Could you check a few things on this model? Use its own coordinates, in mm. A direction names the side the tool comes from. Round coordinates to 2 decimals unless told otherwise and drop trailing zeros. Write each loop counter-clockwise with the first axis right and the second up, starting at its lowest first coordinate (ties: lowest second). Pieces come first, ordered by that corner, then holes.
```python
from build123d import *

# Parameters (mm, degrees)
SKETCH1_R               = 0.6
FINGER_PIP_BODY_DEPTH   = 2
FINGER_PIP_CONTOURING_R = 2


with BuildPart() as part:
    # Sketch1 → Finger PIP Body (new body)
    with BuildSketch(Plane.XY):
        with BuildLine():
            Line((0, 6.5), (0, 33.5))
            add(Edge.make_bspline(
                [(0, 33.5), (3.125, 33.9), (6.25, 33.5)],
                knots=[0, 0, 0, 1, 1, 1], degree=2))
            Line((6.25, 33.5), (6.25, 35.5))
            add(Edge.make_bspline(
                [(0, 35.5), (3.125, 35.1), (6.25, 35.5)],
                knots=[0, 0, 0, 1, 1, 1], degree=2))
            Line((0, 35.5), (0, 40))
            Line((0, 40), (20, 40))
            Line((20, 40), (20, 35.5))
            add(Edge.make_bspline(
                [(20, 35.5), (16.875, 35.1), (13.75, 35.5)],
                knots=[0, 0, 0, 1, 1, 1], degree=2))
            Line((13.75, 35.5), (13.75, 33.5))
            add(Edge.make_bspline(
                [(20, 33.5), (16.875, 33.9), (13.75, 33.5)],
                knots=[0, 0, 0, 1, 1, 1], degree=2))
            Line((20, 33.5), (20, 6.5))
            add(Edge.make_bspline(
                [(20, 6.5), (16.875, 6.1), (13.75, 6.5)],
                knots=[0, 0, 0, 1, 1, 1], degree=2))
            Line((13.75, 6.5), (13.75, 4.5))
            add(Edge.make_bspline(
                [(20, 4.5), (16.875, 4.9), (13.75, 4.5)],
                knots=[0, 0, 0, 1, 1, 1], degree=2))
            Line((20, 4.5), (20, 0))
            Line((20, 0), (0, 0))
            Line((0, 0), (0, 4.5))
            add(Edge.make_bspline(
                [(0, 4.5), (3.125, 4.9), (6.25, 4.5)],
                knots=[0, 0, 0, 1, 1, 1], degree=2))
            Line((6.25, 4.5), (6.25, 6.5))
            add(Edge.make_bspline(
                [(0, 6.5), (3.125, 6.1), (6.25, 6.5)],
                knots=[0, 0, 0, 1, 1, 1], degree=2))
        make_face()
        with Locations((3, 2.5)):
            Circle(SKETCH1_R, mode=Mode.SUBTRACT)
        with Locations((5, 9.5)):
            Circle(SKETCH1_R, mode=Mode.SUBTRACT)
        with Locations((5, 30.5)):
            Circle(SKETCH1_R, mode=Mode.SUBTRACT)
        with Locations((3, 37.5)):
            Circle(SKETCH1_R, mode=Mode.SUBTRACT)
        with Locations((17, 37.5)):
            Circle(SKETCH1_R, mode=Mode.SUBTRACT)
        with Locations((15, 30.5)):
            Circle(SKETCH1_R, mode=Mode.SUBTRACT)
        with Locations((15, 9.5)):
            Circle(SKETCH1_R, mode=Mode.SUBTRACT)
        with Locations((17, 2.5)):
            Circle(SKETCH1_R, mode=Mode.SUBTRACT)
    extrude(amount=FINGER_PIP_BODY_DEPTH)

    # Finger PIP Contouring
    finger_pip_contouring_edges = [part.edges().sort_by_distance(p)[0] for p in [
        (0, 40, 1),
        (20, 40, 1),
        (20, 0, 1),
        (0, 0, 1),
    ]]
    fillet(finger_pip_contouring_edges, radius=FINGER_PIP_CONTOURING_R)


solid = part.part
```
Q1. If I drill on L1, parallel to X at y = 37.5, z = 1.15; L2, parallel to Y at x = 17, z = 1.1; L3, parallel to Y at x = 5.25, z = 0.65, over which ranges is the centre line in solid material (lowest first)?
Q2. Imagine slicing it at B-B, the plane x = 15. Count the separate pieces of the cut face and the enclosed holes in it, then the cut area to 3 significant figures.
Q3. I'm going to push flat-ended pins straight in: pin 1 Ø10 at (x, y) = (10.5, 5) entering from -Z; pin 2 Ø1.1 at (x, y) = (3, 2.5) entering from -Z. Where does each tip first touch, or does it pass through?
Q4. Imagine slicing it at A-A, the plane y = 9.5. Write out the boundary of the cut face in (x, z), then the cut area to 3 significant figures.
Q5. We'd pull the mould along Y, two halves only. Please class faces 1 (the flat face through (0, 20, 1)), 2 (the cylindrical face through (14.922, 31.095, 0.986)), 3 (the flat face through (10, 0, 1)): pulls with the +Y half, pulls with the -Y half, needs draft (parallel to the pull), parting line crosses it, or undercut.
Q6. On a 3-axis mill with a long thin cutter (end or side, diameter ignored), from which of +Z, -Z, +X, -X, +Y, -Y can I reach the whole of each face in a straight line? I mean faces 4 (the flat face through (13.75, 35, 1)), 5 (the flat face through (10, 20, 2)). Say none if no direction works.
Results found:
1. L1: x = 0 to 2.4, 3.6 to 16.4, 17.6 to 20
1. L2: y = 0 to 1.9, 3.1 to 4.7, 6.3 to 33.7, 35.3 to 36.9, 38.1 to 40
1. L3: y = 0 to 4.61, 6.39 to 8.95, 10.05 to 29.95, 31.05 to 33.61, 35.39 to 40
2. separate pieces: 5
2. enclosed holes: 0
2. area: 68.2 mm2
3. pin 1: stops at z = 0
3. pin 2: passes through
4. outline: (0, 0) - (4.4, 0) - (4.4, 2) - (0, 2) - close; (5.6, 0) - (14.4, 0) - (14.4, 2) - (5.6, 2) - close; (15.6, 0) - (20, 0) - (20, 2) - (15.6, 2) - close
4. area: 35.2 mm2
5. face 1: needs draft
5. face 2: undercut
5. face 3: pulls with the -Y half
6. face 4: +Z, -Z
6. face 5: +Z, +X, -X, +Y, -Y
